```python
from build123d import *

# Parameters (mm, degrees)
SKETCH1_W           = 30
SKETCH1_H           = 30
BOSS_EXTRUDE1_DEPTH = 20
SKETCH2_R           = 2
SKETCH2_R_2         = 1.25
CUT_EXTRUDE1_DEPTH  = 20


with BuildPart() as part:
    # Sketch1 → Boss-Extrude1 (new body)
    with BuildSketch(Plane(origin=(0, 0, 0), x_dir=(1, 0, 0), z_dir=(0, 1, 0))):
        with Locations((15, 15)):
            Rectangle(SKETCH1_W, SKETCH1_H)
    extrude(amount=BOSS_EXTRUDE1_DEPTH)

    # Sketch2 → Cut-Extrude1 (cut)
    with BuildSketch(Plane(origin=(0, 20, 0), x_dir=(1, 0, 0), z_dir=(0, 1, 0))):
        with Locations((5, 25)):
            Circle(SKETCH2_R)
        with Locations((5, 5)):
            Circle(SKETCH2_R)
        with Locations((26, 5)):
            Circle(SKETCH2_R)
        with Locations((26, 25)):
            Circle(SKETCH2_R)
        with Locations((15, 15)):
            Circle(SKETCH2_R_2)
    extrude(amount=-CUT_EXTRUDE1_DEPTH, mode=Mode.SUBTRACT)


solid = part.part
```
Input: part model. Units: mm. Frame: model coordinates. Round coordinates to 2 decimals unless told otherwise and drop trailing zeros. Loops run counter-clockwise (first coordinate to the right, second up) from the corner with the lowest first, then second, coordinate; pieces in that order, holes last. Notation, with made-up numbers: (77, 83) -> (116, 83) arc R11 ccw to (116, 99) -> close; hole circle Ø8 at (89, 27). An arc over 180 degrees is marked (long way). One line per item, written item: value.
(1) Section C-C (y = 6.75). Return the cut outline in (x, z), plus the area to 3 significant figures.
Geometry check:
outline: (0, -30) -> (30, -30) -> (30, 0) -> (0, 0) -> close; hole circle Ø4 at (5, -25); hole circle Ø4 at (5, -5); hole circle Ø2.5 at (15, -15); hole circle Ø4 at (26, -25); hole circle Ø4 at (26, -5)
area: 845 mm2
(2) Section D-D (x = 15). Return the cut outline in (y, z).
Geometry check:
outline: (0, -30) -> (20, -30) -> (20, -16.25) -> (0, -16.25) -> close; (0, -13.75) -> (20, -13.75) -> (20, 0) -> (0, 0) -> close
(3) Section A-A (x = 5). Return the cut outline in (y, z).
Geometry check:
outline: (0, -30) -> (20, -30) -> (20, -27) -> (0, -27) -> close; (0, -23) -> (20, -23) -> (20, -7) -> (0, -7) -> close; (0, -3) -> (20, -3) -> (20, 0) -> (0, 0) -> close
(4) Mould query, pull axis Z, two halves, no side actions, for faces 1 (the face through (14.079, 10.14, -15.845)), 2 (the face through (15, 10, 0)), 3 (the face through (15, 10, -30)). Classes: pulls with the +Z half, pulls with the -Z half, needs draft (parallel to the pull), parting line crosses it, or undercut.
Geometry check:
face 1: undercut
face 2: pulls with the +Z half
face 3: pulls with the -Z half
(5) Material intervals for line 1 (Z direction, x = 26, y = 11); line 2 (X direction, y = 8.5, z = -25); line 3 (X direction, y = 5, z = -6.5), sorted ascending. Write a range as [from, to].
Geometry check:
line 1: [-30, -27], [-23, -7], [-3, 0]
line 2: [0, 3], [7, 24], [28, 30]
line 3: [0, 3.68], [6.32, 24.68], [27.32, 30]
(6) Section B-B (z = -25). Return the cut outline in (x, y), plus the area to 3 significant figures.
Geometry check:
outline: (0, 0) -> (3, 0) -> (3, 20) -> (0, 20) -> close; (7, 0) -> (24, 0) -> (24, 20) -> (7, 20) -> close; (28, 0) -> (30, 0) -> (30, 20) -> (28, 20) -> close
area: 440 mm2
